Work out the finished part from the listing and answer in its coordinate system (mm). Round coordinates to 2 decimals unless told otherwise and drop trailing zeros. Order: outer loops, then holes, each group sorted by start corner. A loop starts at its lowest first (then second) coordinate and runs counter-clockwise, first axis right, second up. Notation, with made-up numbers: (-21.5, 82) - (9.5, 82) arc R14 cw to (9.5, 106) - close; hole circle Ø6 at (13, 60.25). An arc over 180 degrees is marked (long way). One line per question, with ' | ' between items. Start each with the question number.
Autodesk Inventor part; units mm, degrees
ref_plane "YZ Plane" through (0, 0, 0) normal (1, 0, 0) x (0, 1, 0)
ref_plane "XZ Plane" through (0, 0, 0) normal (0, 1, 0) x (-1, 0, 0)
ref_plane "XY Plane" through (0, 0, 0) normal (0, 0, 1) x (1, 0, 0)
sketch "Sketch1" plane through (0, 0, 0) normal (0, 1, 0) x (-1, 0, 0)
  circle A0 centre (0, 0) radius 25
  dimension "d0" = 50
extrude "Extrusion1" add sketch "Sketch1" along normal blind 30.2
hole "Hole1" at (0, 0, 0) direction (0, 1, 0) diameter 10 depth 5
sketch "Sketch2" plane through (0, 30.2, 0) normal (0, 1, 0) x (1, 0, 0)
  circle A0 centre (0, 0) radius 5
extrude "Extrusion2" add sketch "Sketch2" along normal blind 5
properties part number "stackLightElement" material "Polycarbonate, Clear"
1) Section B-B on x = 0 is taken. Give the vertices of the cut face in (y, z), and give its area (3 significant figures).
2) Section A-A on z = 0 is taken. Give the vertices of the cut face in (x, y), and give its area (3 significant figures).
3) Section C-C on y = 31 is taken. Give the vertices of the cut face in (x, z), and give its area (3 significant figures).
4) Straight lines are drawn through the part: line 1 (Z direction, x = 0, y = 3.1); line 2 (Y direction, x = -22.5, z = -8.5); line 3 (Y direction, x = -0.5, z = 1). For each, find the intervals that lie inside material, in ascending order.
5) Determine the mould class of faces 1 (the flat face through (0, 35.2, 0)), 2 (the cylindrical face through (4.88, 2.54, 1.08)), 3 (the cylindrical face through (-1.08, 32.66, -4.88)), 4 (the flat face through (0, 5, 0)) for opening direction Z: released by +Z, released by -Z, zero draft, split by the parting line, or undercut.
6) Section D-D on y = 19 is taken. Give the vertices of the cut face in (x, z).
7) Flat-ended cylindrical pins translate along their axes: pin 1 (4 mm diameter, centred on y = 4.5, z = 4, fed in from -X); pin 2 (10 mm diameter, centred on y = 4, z = 10.5, fed in from -X); pin 3 (3 mm diameter, centred on y = 17.5, z = 7.5, fed in from +X). Find the tip coordinate at first contact, or state that the pin passes through.
Recorded:
1) outline: (0, -25) - (30.2, -25) - (30.2, -5) - (35.2, -5) - (35.2, 5) - (30.2, 5) - (30.2, 25) - (0, 25) - (0, 5) - (5, 5) - (5, -5) - (0, -5) - close | area: 1,510 mm²
2) outline: (-25, 0) - (-5, 0) - (-5, 5) - (5, 5) - (5, 0) - (25, 0) - (25, 30.2) - (5, 30.2) - (5, 35.2) - (-5, 35.2) - (-5, 30.2) - (-25, 30.2) - close | area: 1,510 mm²
3) outline: circle Ø10 at (0, 0) | area: 78.5 mm²
4) line 1: z = -25 to -5, 5 to 25 | line 2: y = 0 to 30.2 | line 3: y = 5 to 35.2
5) face 1: zero draft | face 2: undercut | face 3: split by the parting line | face 4: undercut
6) outline: circle Ø50 at (0, 0)
7) pin 1: stops at x = -24.92 | pin 2: stops at x = -24.39 | pin 3: stops at x = 24.27
